```python
from build123d import *

# Parameters (mm, degrees)
SKETCH_1_W          = 15.8
SKETCH_1_H          = 7.8
EXTRUDE_2_DEPTH     = 9.6
SKETCH_2_R          = 2.106660513
EXTRUDE_3_DEPTH     = 1.7
SKETCH_3_R          = 2.5
CUT_EXTRUDE_1_DEPTH = 1.8


with BuildPart() as part:
    # Эскиз1 → Бобышка-Вытянуть2 (new body)
    with BuildSketch(Plane(origin=(0, 0, 0), x_dir=(1, 0, 0), z_dir=(0, 1, 0))):
        with Locations((7.9, 3.9)):
            Rectangle(SKETCH_1_W, SKETCH_1_H)
    extrude(amount=EXTRUDE_2_DEPTH)

    # Эскиз2 → Бобышка-Вытянуть3 (add)
    with BuildSketch(Plane(origin=(0, 9.6, 0), x_dir=(1, 0, 0), z_dir=(0, 1, 0))):
        with Locations((3.9, 3.9)):
            Circle(SKETCH_2_R)
        with Locations((11.9, 3.9)):
            Circle(SKETCH_2_R)
    extrude(amount=EXTRUDE_3_DEPTH)

    # Эскиз3 → Вырез-Вытянуть1 (cut)
    with BuildSketch(Plane.XZ):
        with Locations((11.9, -3.9)):
            Circle(SKETCH_3_R)
        with Locations((3.9, -3.9)):
            Circle(SKETCH_3_R)
    extrude(amount=-CUT_EXTRUDE_1_DEPTH, mode=Mode.SUBTRACT)


solid = part.part
```
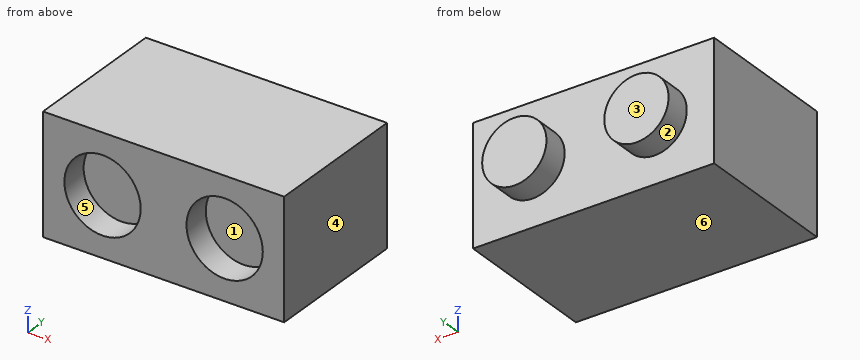
Part model, mm, in its own coordinate system. Face numbers are marked on the shaded views. A direction names the side the tool comes from. Round coordinates to 2 decimals unless told otherwise and drop trailing zeros. Loops run counter-clockwise (first coordinate to the right, second up) from the corner with the lowest first, then second, coordinate; pieces in that order, holes last.
Item 1: Cut at C-C, the plane y = 10.5. Give the cut face in (x, z).
Item 2: Drill centre lines: line 1 (Z direction, x = 3.9, y = 0.9); line 2 (X direction, y = 11, z = -4); line 3 (Y direction, x = 4.5, z = -3.75). Where is each one in solid material? Low to high.
Item 3: Drop flat-ended pins along their axis: P1, Ø1.5, axis at x = 2.5, z = -3, coming from the -Y side; P2, Ø1.5, axis at x = 9, z = -3.5, coming from the +Y side. Give the stop position or say it passes through.
Item 4: Mould opens along Z. For the marked faces 4, 5 and 6 say: +Z half, -Z half, draft (parallel to the pull), parting line (faces both ways), or undercut.
Item 5: Cut at D-D, the plane z = -3. Give the cut face in (x, y).
Item 6: Cut at B-B, the plane z = -3.9. Give the cut face in (x, y).
Item 7: Cut at A-A, the plane x = 11.9. Give the cut face in (y, z).
Item 8: 3-axis set-ups, long thin cutter, end or side, ignore diameter. For the marked faces 1, 2 and 3: which of +Z, -Z, +X, -X, +Y, -Y reach the whole face in a straight line?
A:
1. outline: circle Ø4.21 at (3.9, -3.9); circle Ø4.21 at (11.9, -3.9)
2. line 1: z = -7.8 to -6.4, -1.4 to 0
2. line 2: x = 1.8 to 6, 9.8 to 14
2. line 3: y = 1.8 to 11.3
3. P1: stops at y = 1.8
3. P2: stops at y = 9.6
4. face 4: draft
4. face 5: undercut
4. face 6: -Z half
5. outline: (0, 0) - (1.57, 0) - (1.57, 1.8) - (6.23, 1.8) - (6.23, 0) - (9.57, 0) - (9.57, 1.8) - (14.23, 1.8) - (14.23, 0) - (15.8, 0) - (15.8, 9.6) - (13.8, 9.6) - (13.8, 11.3) - (10, 11.3) - (10, 9.6) - (5.8, 9.6) - (5.8, 11.3) - (2, 11.3) - (2, 9.6) - (0, 9.6) - close
6. outline: (0, 0) - (1.4, 0) - (1.4, 1.8) - (6.4, 1.8) - (6.4, 0) - (9.4, 0) - (9.4, 1.8) - (14.4, 1.8) - (14.4, 0) - (15.8, 0) - (15.8, 9.6) - (14.01, 9.6) - (14.01, 11.3) - (9.79, 11.3) - (9.79, 9.6) - (6.01, 9.6) - (6.01, 11.3) - (1.79, 11.3) - (1.79, 9.6) - (0, 9.6) - close
7. outline: (0, -7.8) - (9.6, -7.8) - (9.6, -6.01) - (11.3, -6.01) - (11.3, -1.79) - (9.6, -1.79) - (9.6, 0) - (0, 0) - (0, -1.4) - (1.8, -1.4) - (1.8, -6.4) - (0, -6.4) - close
8. face 1: -Y
8. face 2: +Y
8. face 3: +Z, -Z, +X, -X, +Y
